For this review, use the dimensioned drawing (mm, ordinates from the lowest corner) and the shaded views. Coordinates: 2 decimals unless noted, no trailing zeros. Loops run counter-clockwise (first coordinate to the right, second up) from the corner with the lowest first, then second, coordinate; pieces in that order, holes last. Notation, with made-up numbers: M 12.25,22 L 44.25,22 A18 ccw 44.25,27 Z; hole C -29,56.5 d4. An arc over 180 degrees is marked long. One line per item, written item: value.
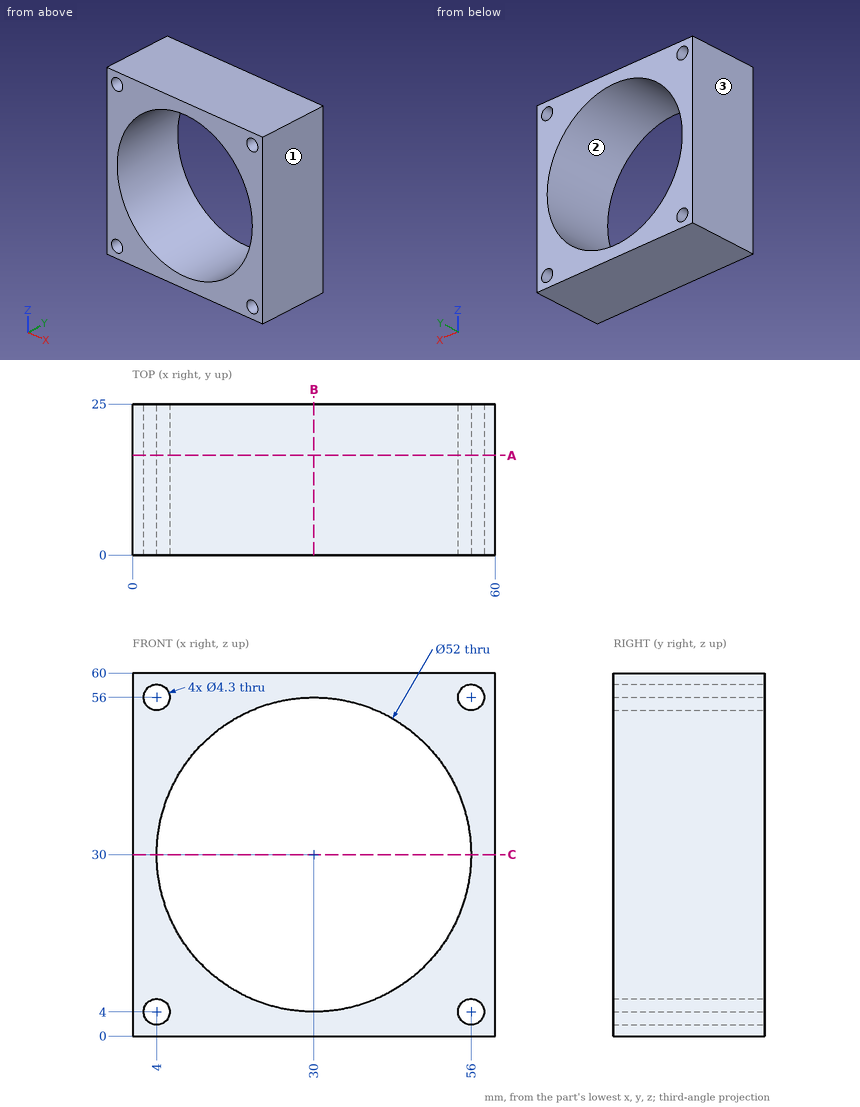
(1) Draft analysis for pull direction X (two halves, no side actions). For the marked faces 1, 2 and 3, state which applies: pulls with the +X half, pulls with the -X half, needs draft (parallel to the pull), parting line crosses it, or undercut.
Checks:
face 1: pulls with the +X half
face 2: undercut
face 3: pulls with the -X half
(2) Add section B-B on x = 30. State the section outline as (y, z) points, then the cut area to 3 significant figures.
Checks:
outline: M 0,0 L 25,0 L 25,4 L 0,4 Z; M 0,56 L 25,56 L 25,60 L 0,60 Z
area: 200 mm^2
(3) Add section A-A on y = 16.5. State the section outline as (x, z) points, then the cut area to 3 significant figures.
Checks:
outline: M 0,0 L 60,0 L 60,60 L 0,60 Z; hole C 4,4 d4.3; hole C 4,56 d4.3; hole C 30,30 d52; hole C 56,4 d4.3; hole C 56,56 d4.3
area: 1,420 mm^2
(4) Insertion check: pin 1 Ø8 at (x, z) = (46, 20.5) entering from -Y (3 decimals). The pin has a flat end and moves straight along its axis. Give the tip position at first contact, or say it passes through.
Checks:
pin 1: through
(5) Add section C-C on z = 30. State the section outline as (x, y) points.
Checks:
outline: M 0,0 L 4,0 L 4,25 L 0,25 Z; M 56,0 L 60,0 L 60,25 L 56,25 Z
(6) To check wall thickness, follow L1, parallel to Z at x = 30, y = 19.25; L2, parallel to X at y = 13.75, z = 6.5; L3, parallel to X at y = 23.5, z = 37. State the ranges of each line that lie inside material, in increasing order. Write a range as [from, to].
Checks:
L1: [0, 4], [56, 60]
L2: [0, 18.88], [41.12, 60]
L3: [0, 4.96], [55.04, 60]
